from build123d import *

# Parameters (mm, degrees)
SKETCH1_W                    = 25.4
SKETCH1_H                    = 50.8
SKETCH1_W_2                  = 19.05
SKETCH1_H_2                  = 44.45
BOSS_EXTRUDE1_DEPTH          = 19.05
F_10_0_1935_DIAMETER_HOLE1_D = 4.9149
F_10_32_TAPPED_HOLE1_D       = 4.0386


with BuildPart() as part:
    # Sketch1 → Boss-Extrude1 (new, symmetric)
    with BuildSketch(Plane.XY):
        Rectangle(SKETCH1_W, SKETCH1_H)
        Rectangle(SKETCH1_W_2, SKETCH1_H_2, mode=Mode.SUBTRACT)
    extrude(amount=BOSS_EXTRUDE1_DEPTH, both=True)

    # #10 (0.1935) Diameter Hole1 (through all)
    with Locations(Plane(origin=(0, 25.4, 0), x_dir=(1, 0, 0), z_dir=(0, 1, 0))):
        with Locations((-4.7625, -12.7), (-4.7625, 12.7)):
            Hole(F_10_0_1935_DIAMETER_HOLE1_D / 2)

    # #10-32 Tapped Hole1 (through all)
    with Locations(Plane.ZY.offset(12.7)):
        with Locations((-12.7, -12.7), (12.7, -12.7), (0, 12.7)):
            Hole(F_10_32_TAPPED_HOLE1_D / 2)


solid = part.part
The listing builds one solid part. Answer for the finished solid, in the listing's coordinates (mm). A direction names the side the tool comes from. Give positions to 0.01 mm unless a question says otherwise; leave off trailing zeros. Loops run counter-clockwise (first coordinate to the right, second up) from the corner with the lowest first, then second, coordinate; pieces in that order, holes last. Notation, with made-up numbers: (-13, 73) - (37, 73) arc R24 cw to (37, 87) - close; hole circle Ø4 at (-36.5, 36). An arc over 180 degrees is marked (long way). Use one line per item in the form item = value.
1. Which of the six approach directions +Z, -Z, +X, -X, +Y, -Y give full straight-line access (tool end or side, diameter ignored) to faces 1 (the face through (0, 22.225, 0)), 2 (the face through (11.135, -10.698, 12.963))?
Calculated:
face_1 = +Z, -Z
face_2 = +X, -X
2. The mould has two halves that part along Y. Classify faces 3 (the face through (0, -25.4, 0)), 4 (the face through (0, -22.225, 0)), 5 (the face through (-4.23, 23.79, 15.1)): pulls with the +Y half, pulls with the -Y half, needs draft (parallel to the pull), parting line crosses it, or undercut.
Calculated:
face_3 = pulls with the -Y half
face_4 = undercut
face_5 = needs draft
3. Section A-A on x = -0.5 is taken. Give the vertices of the cut face in (y, z) (3 decimals).
Calculated:
outline = (-25.4, -19.05) - (-22.225, -19.05) - (-22.225, 19.05) - (-25.4, 19.05) - close; (22.225, -19.05) - (25.4, -19.05) - (25.4, 19.05) - (22.225, 19.05) - close
4. Given pin 1 Ø6.5 at (y, z) = (12.7, 0) entering from +X; pin 2 Ø4.5 at (x, z) = (-4.76, 12.7) entering from -Y, each flat-ended and moving along its own axis, determine where each tip first touches the part or whether it passes through.
Calculated:
pin_1 = 12.7
pin_2 = through
5. Section B-B on y = -12.7 is taken. Give the vertices of the cut face in (x, z) (3 decimals).
Calculated:
outline = (-12.7, -19.05) - (-9.525, -19.05) - (-9.525, -14.719) - (-12.7, -14.719) - close; (-12.7, -10.681) - (-9.525, -10.681) - (-9.525, 10.681) - (-12.7, 10.681) - close; (-12.7, 14.719) - (-9.525, 14.719) - (-9.525, 19.05) - (-12.7, 19.05) - close; (9.525, -19.05) - (12.7, -19.05) - (12.7, -14.719) - (9.525, -14.719) - close; (9.525, -10.681) - (12.7, -10.681) - (12.7, 10.681) - (9.525, 10.681) - close; (9.525, 14.719) - (12.7, 14.719) - (12.7, 19.05) - (9.525, 19.05) - close
6. Section C-C on z = -12.7 is taken. Give the vertices of the cut face in (x, y) (3 decimals), then the cut area to 3 significant figures.
Calculated:
outline = (-12.7, -25.4) - (-7.22, -25.4) - (-7.22, -22.225) - (-9.525, -22.225) - (-9.525, -14.719) - (-12.7, -14.719) - close; (-12.7, -10.681) - (-9.525, -10.681) - (-9.525, 22.225) - (-7.22, 22.225) - (-7.22, 25.4) - (-12.7, 25.4) - close; (-2.305, -25.4) - (12.7, -25.4) - (12.7, -14.719) - (9.525, -14.719) - (9.525, -22.225) - (-2.305, -22.225) - close; (-2.305, 22.225) - (9.525, 22.225) - (9.525, -10.681) - (12.7, -10.681) - (12.7, 25.4) - (-2.305, 25.4) - close
area = 387 mm^2
7. Section D-D on x = -10.5 is taken. Give the vertices of the cut face in (y, z).
Calculated:
outline = (-25.4, -19.05) - (25.4, -19.05) - (25.4, 19.05) - (-25.4, 19.05) - close; hole circle Ø4.04 at (-12.7, -12.7); hole circle Ø4.04 at (-12.7, 12.7); hole circle Ø4.04 at (12.7, 0)
8. Find the intervals of material crossed by line 1 along X through (y, z) = (3, 5.5) (3 decimals); line 2 along Y through (x, z) = (8.5, 9) (3 decimals); line 3 along Y through (x, z) = (-10.55, 0), in increasing order. Write a range as [from, to].
Calculated:
line_1 = [-12.7, -9.525], [9.525, 12.7]
line_2 = [-25.4, -22.225], [22.225, 25.4]
line_3 = [-25.4, 10.68], [14.72, 25.4]
